Can you work these out from the drawing? Everything is in mm from the part's minimum corner. A direction names the side the tool comes from. Round coordinates to 2 decimals unless told otherwise and drop trailing zeros. Order: outer loops, then holes, each group sorted by start corner. A loop starts at its lowest first (then second) coordinate and runs counter-clockwise, first axis right, second up. Notation, with made-up numbers: M 75.5,-37.75 L 117.5,-37.75 A21 cw 117.5,0.25 Z; hole C 22.5,54 d1. An arc over 180 degrees is marked long. Answer as a JSON object with one key per item and string values. Group by question number.
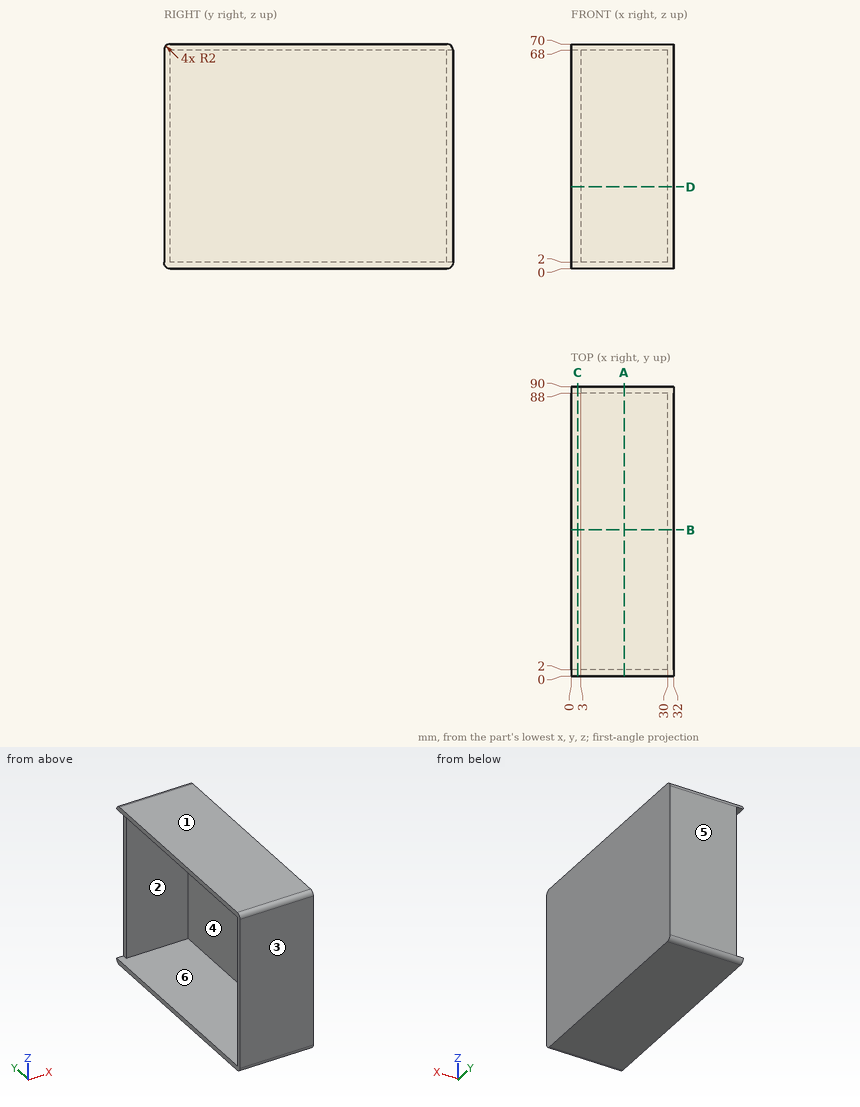
Item 1: Suppose I cut it at D-D, the plane z = 25.5. Write out the boundary of the cut face in (x, y), and give its area (3 significant figures).
Item 2: Suppose I cut it at A-A, the plane x = 16.5. Write out the boundary of the cut face in (y, z), and give its area (3 significant figures).
Item 3: I need wall thicknesses on line 1 (Z direction, x = 20, y = 46); line 2 (Y direction, x = 21.5, z = 38); line 3 (X direction, y = 6.5, z = 33). Which ranges of each line are inside material? Lowest first, please.
Item 4: Suppose I cut it at C-C, the plane x = 2. Write out the boundary of the cut face in (y, z), and give its area (3 significant figures).
Item 5: Suppose I cut it at B-B, the plane y = 45.5. Write out the boundary of the cut face in (x, z).
Item 6: On a 3-axis mill with a long thin cutter (end or side, diameter ignored), from which of +Z, -Z, +X, -X, +Y, -Y can I reach the whole of each face in a straight line? I mean the marked faces 5 and 6. Say none if no direction works.
Item 7: I'm going to push flat-ended pins straight in: pin 1 Ø0.6 at (y, z) = (89, 41) entering from -X; pin 2 Ø1.5 at (y, z) = (44, 26) entering from -X. Where does each tip first touch, or does it pass through?
Item 8: If we mould it in two halves opening along Y, with no side actions, what happens to the marked faces 1, 2, 3 and 4? For each: +Y half, -Y half, draft (parallel to the pull), parting line (faces both ways), or undercut.
Computed:
{
 "1": {"outline": "M 0,0 L 32,0 L 32,90 L 3,90 L 3,88 L 30,88 L 30,2 L 0,2 Z", "area": "294 mm^2"},
 "2": {"outline": "M 0,2 A2 ccw 2,0 L 88,0 A2 ccw 90,2 L 90,68 A2 ccw 88,70 L 2,70 A2 ccw 0,68 Z; hole M 2,2 L 88,2 L 88,68 L 2,68 Z", "area": "621 mm^2"},
 "3": {"line 1": "z = 0 to 2, 68 to 70", "line 2": "y = 0 to 2, 88 to 90", "line 3": "x = 30 to 32"},
 "4": {"outline": "M 0,2 A2 ccw 2,0 L 88,0 A2 ccw 90,2 L 2,2 L 2,68 L 90,68 A2 ccw 88,70 L 2,70 A2 ccw 0,68 Z", "area": "489 mm^2"},
 "5": {"outline": "M 0,0 L 32,0 L 32,70 L 0,70 L 0,68 L 30,68 L 30,2 L 0,2 Z"},
 "6": {"face 5": "+Z, -Z, +X, -X, +Y", "face 6": "-X"},
 "7": {"pin 1": "stops at x = 3", "pin 2": "stops at x = 30"},
 "8": {"face 1": "draft", "face 2": "undercut", "face 3": "-Y half", "face 4": "undercut"}
}
